Here's the drawing with two shaded views (mm, measured from the low corner). I have some questions. A direction names the side the tool comes from. Round coordinates to 2 decimals unless told otherwise and drop trailing zeros. Loops run counter-clockwise (first coordinate to the right, second up) from the corner with the lowest first, then second, coordinate; pieces in that order, holes last.
(1) If I drill on line 1 along X through (y, z) = (0.85, 27.5); line 2 along X through (y, z) = (27, 12); line 3 along Z through (x, y) = (4, 1), over which ranges is the centre line in solid material (lowest first)?
(2) Which directions (+Z, -Z, +X, -X, +Y, -Y) give clear straight access to the entire face, cutting with the end or side of a thin tool? Please do the marked faces 1, 2, 3 and 4.
(3) I want a section at A-A on z = 27.5. Write out the boundary of the cut face in (x, y).
(4) I want a section at D-D on z = 15.5. Write out the boundary of the cut face in (x, y), plus the area to 3 significant figures.
(5) I want a section at B-B on y = 22.5. Write out the boundary of the cut face in (x, z).
(6) I want a section at C-C on x = 30.5. Write out the boundary of the cut face in (y, z), plus the area to 4 significant figures.
(7) Will these pins go through, and if not, where does the flat tip stop? pin 1 Ø9.5 at (x, z) = (18.5, 11) entering from +Y; pin 2 Ø10 at (x, z) = (16, 26) entering from -Y; pin 3 Ø3.5 at (x, z) = (34.5, 27.5) entering from -Y; pin 4 Ø1.5 at (x, y) = (34, 7.5) entering from +Z.
(8) Thinking about a two-plate mould opening in X: for the marked faces 5, 6 and 7, which applies, released by +X, released by -X, zero draft, split by the parting line, or undercut?
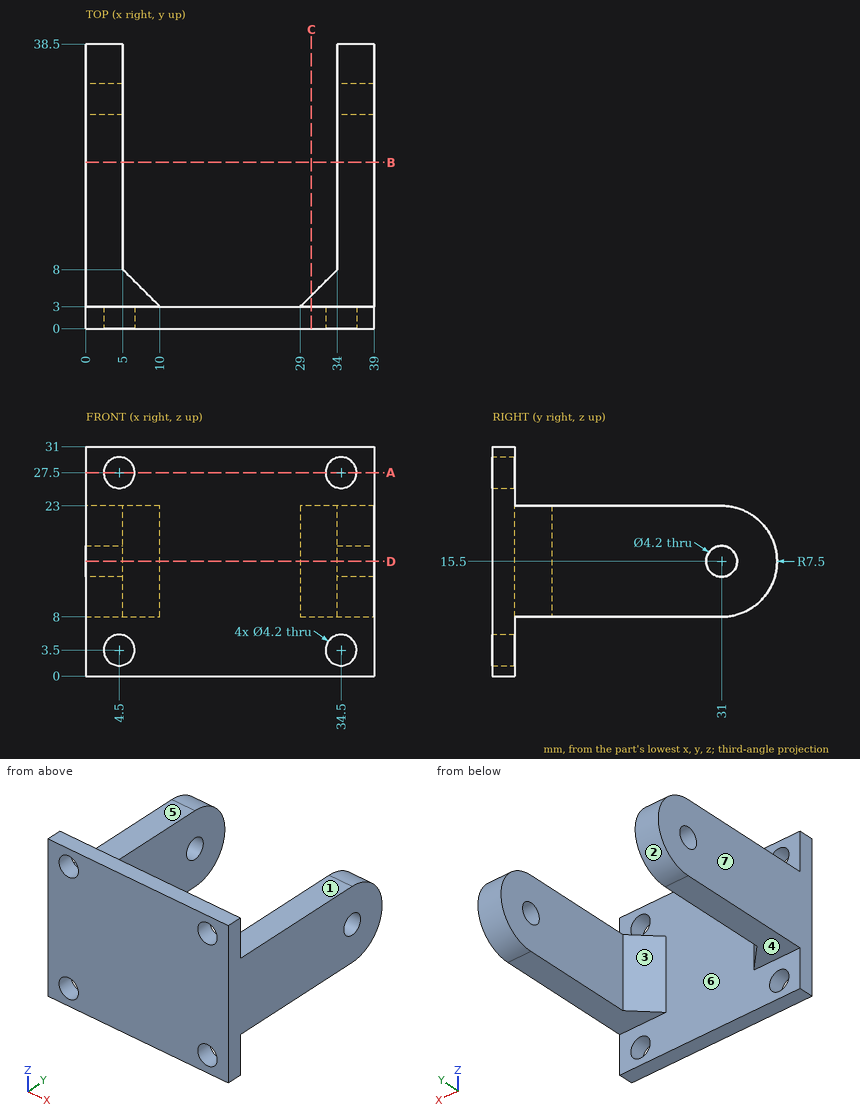
Filled sheet:
1. line 1: x = 0 to 2.4, 6.6 to 32.4, 36.6 to 39
1. line 2: x = 0 to 5, 34 to 39
1. line 3: z = 0 to 1.46, 5.54 to 25.46, 29.54 to 31
2. face 1: +Z, +X, -X, +Y
2. face 2: +X, -X, +Y
2. face 3: +Z, -Z, +Y
2. face 4: -Z, +X, -X, +Y
3. outline: (0, 0) - (2.4, 0) - (2.4, 3) - (0, 3) - close; (6.6, 0) - (32.4, 0) - (32.4, 3) - (6.6, 3) - close; (36.6, 0) - (39, 0) - (39, 3) - (36.6, 3) - close
4. outline: (0, 0) - (39, 0) - (39, 28.9) - (34, 28.9) - (34, 8) - (29, 3) - (10, 3) - (5, 8) - (5, 28.9) - (0, 28.9) - close; (0, 33.1) - (5, 33.1) - (5, 38.5) - (0, 38.5) - close; (34, 33.1) - (39, 33.1) - (39, 38.5) - (34, 38.5) - close
4. area: 455 mm2
5. outline: (0, 8) - (5, 8) - (5, 23) - (0, 23) - close; (34, 8) - (39, 8) - (39, 23) - (34, 23) - close
6. outline: (0, 0) - (3, 0) - (3, 8) - (4.5, 8) - (4.5, 23) - (3, 23) - (3, 31) - (0, 31) - close
6. area: 115.5 mm2
7. pin 1: stops at y = 3
7. pin 2: stops at y = 0
7. pin 3: passes through
7. pin 4: stops at z = 23
8. face 5: zero draft
8. face 6: undercut
8. face 7: released by -X
